Could you check a few things on this model? Use its own coordinates, in mm. A direction names the side the tool comes from. Round coordinates to 2 decimals unless told otherwise and drop trailing zeros. Write each loop counter-clockwise with the first axis right and the second up, starting at its lowest first coordinate (ties: lowest second). Pieces come first, ordered by that corner, then holes. Notation, with made-up numbers: M 37.5,-29 L 43.5,-29 A29 ccw 43.5,-8 Z; hole C 85.25,44.25 d2. An arc over 180 degrees is marked long. One line per item, written item: value. Start each with the question number.
(1) Thinking about a two-plate mould opening in X: for faces 5 (the face through (-4, -17, 7.4)), 6 (the face through (-1.45, -17, 7)), 7 (the face through (-10.79, 10.99, 6.11)), which applies, released by +X, released by -X, zero draft, split by the parting line, or undercut?
(2) Which directions (+Z, -Z, +X, -X, +Y, -Y) give clear straight access to the entire face, cutting with the end or side of a thin tool? Please do faces 1 (the face through (9, 0, 0)), 2 (the face through (4, -17, -7.4)), 3 (the face through (4, -17, 7.4)), 4 (the face through (-1.45, -17, -7)).
(3) I want a section at D-D on x = -8.75. Please give me the cut outline in (y, z), and give its area (3 significant figures).
(4) I'm going to push flat-ended pins straight in: pin 1 Ø5.5 at (x, y) = (-3, -18) entering from -Z; pin 2 Ø1.4 at (x, y) = (2.5, -16.5) entering from +Z; pin 3 Ø2 at (y, z) = (-5, -6.5) entering from +X. Where does each tip first touch, or does it pass through?
(5) I want a section at C-C on y = 11. Please give me the cut outline in (x, z).
(6) I want a section at B-B on z = 10.5. Please give me the cut outline in (x, y).
(7) I want a section at A-A on y = -17. Please give me the cut outline in (x, z), and give its area (3 significant figures).
(8) If I drill on L1, parallel to X at y = 14.1, z = 0; L2, parallel to Y at x = 4.75, z = 3.5; L3, parallel to X at y = -9.5, z = -2, over which ranges is the centre line in solid material (lowest first)?
```python
from build123d import *
from build123d.topology import SkipClean

# Parameters (mm, degrees)
SKETCH_1_R      = 11
EXTRUDE_1_DEPTH = 10
EXTRUDE_2_DEPTH = 2
SKETCH_3_R      = 12.4
EXTRUDE_3_DEPTH = 2
SKETCH_5_R      = 11.264641855
SKETCH_5_R_2    = 9.25178024
EXTRUDE_4_DEPTH = 0.2
EXTRUDE_START   = 12.7
SKETCH_6_W      = 14
SKETCH_6_H      = 16.970562748
EXTRUDE_5_DEPTH = 12.7
SKETCH_7_W      = 4.8
SKETCH_7_H      = 0.8
EXTRUDE_6_DEPTH = 8


with BuildPart() as part:
    # 草图1 → 凸台-拉伸1 (new body)
    with BuildSketch(Plane(origin=(0, 0, 0), x_dir=(1, 0, 0), z_dir=(0, 1, 0))):
        with Locations(Location((0, 0, 0), (0, 0, 270))):
            Circle(SKETCH_1_R)
    extrude(amount=EXTRUDE_1_DEPTH)

    # 草图2 → 凸台-拉伸2 (add)
    with BuildSketch(Plane(origin=(0, 10, 0), x_dir=(1, 0, 0), z_dir=(0, 1, 0))):
        Polygon((7.159143338, -12.4), (14.318286676, 0), (7.159143338, 12.4), (-7.159143338, 12.4), (-14.318286676, 0), (-7.159143338, -12.4), align=None)
    extrude(amount=EXTRUDE_2_DEPTH)

    # 草图3 → 凸台-拉伸3 (add)
    with BuildSketch(Plane(origin=(0, 12, 0), x_dir=(1, 0, 0), z_dir=(0, 1, 0))):
        with Locations(Location((0, 0, 0), (0, 0, 270))):
            Circle(SKETCH_3_R)
    extrude(amount=EXTRUDE_3_DEPTH)

    # 草图5 → 凸台-拉伸4 (add)
    # profile 1 of 3: a face of its own
    with BuildSketch(Plane(origin=(0, 14, 0), x_dir=(1, 0, 0), z_dir=(0, 1, 0))):
        with Locations(Location((0, 0, 0), (0, 0, 270))):
            Circle(SKETCH_5_R)
        with Locations(Location((0, 0, 0), (0, 0, 270))):
            Circle(SKETCH_5_R_2, mode=Mode.SUBTRACT)
    # profile 2 of 3: a face of its own
    with BuildSketch(Plane(origin=(0, 14, 0), x_dir=(1, 0, 0), z_dir=(0, 1, 0))):
        with BuildLine():
            add(Edge.make_bspline(
                [(-4.531930976, 3.945494062), (-4.931928742, 3.77750387), (-5.311682001, 2.960342277), (-5.991141543, 1.949169031), (-6.396271783, 0.524296362), (-6.537370068, -1.286255496), (-5.840461103, -3.78050422), (-3.973519682, -6.124461985), (-1.238390819, -7.169357291), (1.520794025, -7.173420809), (4.211359131, -6.084158365), (6.086695891, -3.477668911), (6.905357115, -0.367726074), (5.905130942, 2.059620867), (5.028765713, 3.962793153), (3.875298238, 4.041756072), (3.29141668, 3.696344725), (3.048713235, 3.141954909), (3.061357601, 2.526413251), (3.488195445, 2.234620856), (3.679341437, 1.769390855), (4.169012756, 1.362737183), (4.223062658, 0.659416394), (4.515624189, -0.227999974), (4.461264715, -1.369716105), (4.079353431, -2.593948769), (3.30330561, -3.914996189), (1.935894526, -4.815540791), (0.278175009, -5.149155893), (-1.219670545, -5.004826573), (-2.832376043, -4.211829708), (-4.044284214, -2.735827002), (-4.496323869, -0.944601433), (-4.311986077, 0.553939945), (-3.824616639, 1.652646984), (-3.227775265, 2.283187209), (-2.88981713, 2.939912012), (-3.127884309, 3.699186823), (-3.820836776, 4.050553792), (-4.341264245, 4.025569861), (-4.531930976, 3.945494062)],
                knots=[0, 0, 0, 0, 0.023973889, 0.04155419, 0.066468029, 0.100998981, 0.137141746, 0.20193186, 0.251863159, 0.287326725, 0.347456235, 0.39706454, 0.454431749, 0.507559151, 0.538353321, 0.553211894, 0.562961677, 0.572498599, 0.584637384, 0.591443225, 0.598437343, 0.610871675, 0.62326923, 0.634065974, 0.660780987, 0.681865173, 0.702097016, 0.741217122, 0.764094276, 0.791316499, 0.819614085, 0.857637757, 0.888785096, 0.915262001, 0.936720816, 0.951197394, 0.961514557, 0.974340001, 0.988572379, 1, 1, 1, 1], degree=3))
        make_face()
    # profile 3 of 3: a face of its own
    with BuildSketch(Plane(origin=(0, 14, 0), x_dir=(1, 0, 0), z_dir=(0, 1, 0))):
        with BuildLine():
            Line((-0.953053843, 6.387223198), (-0.953053843, 1.620615101))
            ThreePointArc((-0.953053843, 1.620615101), (0.003085924, 0.707999599), (1.047457876, 1.518158555))
            Line((1.047457876, 1.518158555), (1.047457876, 6.387223198))
            ThreePointArc((1.047457876, 6.387223198), (0.047202017, 7.135854771), (-0.953053843, 6.387223198))
        make_face()
    extrude(amount=EXTRUDE_4_DEPTH)

    # 草图6 → 凸台-拉伸5 (add)
    with SkipClean():  # the faces are left unmerged after this step: merging them gives an invalid solid
        with BuildSketch(Plane.XZ.offset(EXTRUDE_START)):
            Rectangle(SKETCH_6_W, SKETCH_6_H)
            with BuildLine():
                Line((-7, 8.485281374), (7, 8.485281374))
                ThreePointArc((7, 8.485281374), (0, 11), (-7, 8.485281374))
            make_face()
            with BuildLine():
                ThreePointArc((-7, -8.485281374), (0, -11), (7, -8.485281374))
                Line((7, -8.485281374), (-7, -8.485281374))
            make_face()
        extrude(amount=-EXTRUDE_5_DEPTH)

    # 草图7 → 凸台-拉伸6 (add)
    with SkipClean():  # the faces are left unmerged after this step: merging them gives an invalid solid
        with BuildSketch(Plane.XZ.offset(12.7)):
            with Locations((3.85, 7)):
                Rectangle(SKETCH_7_W, SKETCH_7_H)
            with Locations((-3.85, 7)):
                Rectangle(SKETCH_7_W, SKETCH_7_H)
            with Locations((3.85, -7)):
                Rectangle(SKETCH_7_W, SKETCH_7_H)
            with Locations((-3.85, -7)):
                Rectangle(SKETCH_7_W, SKETCH_7_H)
        extrude(amount=EXTRUDE_6_DEPTH)


solid = part.part
```
Found:
1. face 5: zero draft
1. face 6: undercut
1. face 7: released by -X
2. face 1: +Z, -Z, +X, -Y
2. face 2: -Z, +X, -X, -Y
2. face 3: +Z, +X, -X, -Y
2. face 4: +Z, -Z, -Y
3. outline: M 0,-6.67 L 10,-6.67 L 10,-9.64 L 12,-9.64 L 12,-8.79 L 14,-8.79 L 14,-7.09 L 14.2,-7.09 L 14.2,-3.01 L 14,-3.01 L 14,3.01 L 14.2,3.01 L 14.2,7.09 L 14,7.09 L 14,8.79 L 12,8.79 L 12,9.64 L 10,9.64 L 10,6.67 L 0,6.67 Z
3. area: 209 mm²
4. pin 1: stops at z = -7.4
4. pin 2: stops at z = 7.4
4. pin 3: stops at x = 7
5. outline: M -14.32,0 L -7.16,-12.4 L 7.16,-12.4 L 14.32,0 L 7.16,12.4 L -7.16,12.4 Z
6. outline: M -8.26,10 L -3.28,10 L -3.28,-12.7 L 3.28,-12.7 L 3.28,10 L 8.26,10 L 8.26,12 L 6.6,12 L 6.6,14 L 4.08,14 L 4.08,14.2 L -4.08,14.2 L -4.08,14 L -6.6,14 L -6.6,12 L -8.26,12 Z
7. outline: M -6.25,-7.4 L -1.45,-7.4 L -1.45,-6.6 L -6.25,-6.6 Z; M -6.25,6.6 L -1.45,6.6 L -1.45,7.4 L -6.25,7.4 Z; M 1.45,-7.4 L 6.25,-7.4 L 6.25,-6.6 L 1.45,-6.6 Z; M 1.45,6.6 L 6.25,6.6 L 6.25,7.4 L 1.45,7.4 Z
7. area: 15.4 mm²
8. L1: x = -11.26 to -9.25, -6.41 to -4.36, 4.41 to 6.53, 9.25 to 11.26
8. L2: y = -12.7 to 14.2
8. L3: x = -7 to 7
